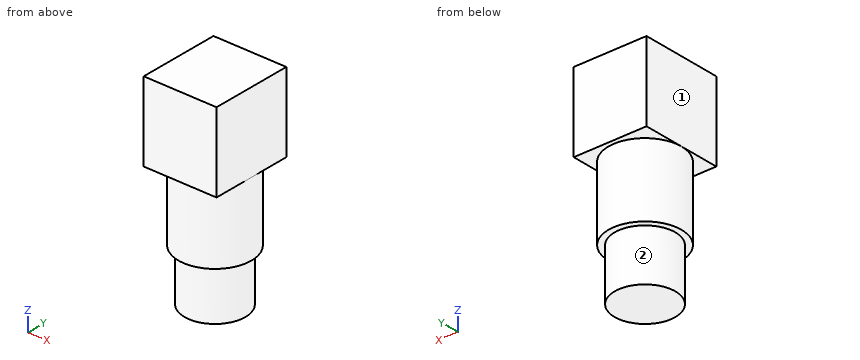
from build123d import *

# Parameters (mm, degrees)
SKETCH003_W             = 12
SKETCH003_H             = 13.4
PAD003_DEPTH            = 13
SKETCH004_R             = 6
PAD004_DEPTH            = 12
SKETCH005_R             = 5
PAD005_DEPTH            = 8.5
BODY002_PLACEMENT_ANGLE = 180


with BuildPart() as part:
    # Sketch003 → Pad003 (new body)
    with BuildSketch(Plane.XY):
        with Locations((6, 6.7)):
            Rectangle(SKETCH003_W, SKETCH003_H)
    extrude(amount=PAD003_DEPTH)

    # Sketch004 (on Face6 of Pad003) → Pad004 (join)
    with BuildSketch(Plane.XY.offset(13)):
        with Locations((6, 6.7)):
            Circle(SKETCH004_R)
    extrude(amount=PAD004_DEPTH)

    # Sketch005 (on Face9 of Pad004) → Pad005 (join)
    with BuildSketch(Plane.XY.offset(25)):
        with Locations((6, 6.7)):
            Circle(SKETCH005_R)
    extrude(amount=PAD005_DEPTH)


with BuildPart() as part_1:
    # Body002 placement: moved
    add(part.part.moved(Location((-6.2, 6.8, -2.4))).rotate(Axis((-6.2, 6.8, -2.4), (1, 0, 0)), BODY002_PLACEMENT_ANGLE))


solid = part_1.part
The model under review builds one solid part; all positions refer to its coordinate system, in mm. Face numbers are marked on the shaded views. A direction names the side the tool comes from. Round coordinates to 2 decimals unless told otherwise and drop trailing zeros. Loops run counter-clockwise (first coordinate to the right, second up) from the corner with the lowest first, then second, coordinate; pieces in that order, holes last. Notation, with made-up numbers: M 57,-8 L 63,-8 A7 cw 63,-4 Z; hole C 44.5,45.25 d8. An arc over 180 degrees is marked long. Answer as a JSON object with one key per item and string values.
Item 1: For line 1 along Z through (x, y) = (-4, 4); line 2 along Z through (x, y) = (-4.25, -6); line 3 along X through (y, z) = (2.5, -25), list the stretches that pass through material, from the lowest coordinate up.
Check sheet entries:
{"line 1": "-27.4 to -2.4", "line 2": "-15.4 to -2.4", "line 3": "-5.7 to 5.3"}
Item 2: We need section A-A, the plane x = -0.2. State the section outline as (y, z) points, and give its area (3 significant figures).
Check sheet entries:
{"outline": "M -6.6,-15.4 L -5.9,-15.4 L -5.9,-27.4 L -4.9,-27.4 L -4.9,-35.9 L 5.1,-35.9 L 5.1,-27.4 L 6.1,-27.4 L 6.1,-15.4 L 6.8,-15.4 L 6.8,-2.4 L -6.6,-2.4 Z", "area": "403 mm2"}
Item 3: We need section B-B, the plane y = 1.25. State the section outline as (x, z) points, and give its area (3 significant figures).
Check sheet entries:
{"outline": "M -6.2,-15.4 L -6.09,-15.4 L -6.09,-27.4 L -5.07,-27.4 L -5.07,-35.9 L 4.67,-35.9 L 4.67,-27.4 L 5.69,-27.4 L 5.69,-15.4 L 5.8,-15.4 L 5.8,-2.4 L -6.2,-2.4 Z", "area": "380 mm2"}
Item 4: We need section C-C, the plane z = -31.5. State the section outline as (x, y) points, and give its area (3 significant figures).
Check sheet entries:
{"outline": "C -0.2,0.1 d10", "area": "78.5 mm2"}
Item 5: Clearance check with flat-ended pins moving along their axes: P1, Ø1.5, axis at y = 3.5, z = -28, coming from the +X side; P2, Ø3, axis at y = 2, z = -19.5, coming from the -X side; P3, Ø1, axis at y = -3.5, z = -22.5, coming from the -X side; P4, Ø3.5, axis at x = -1.5, y = -5, coming from the -Z side. State where each tip first meets the part, or that it passes through.
Check sheet entries:
{"P1": "x = 5.02", "P2": "x = -6.19", "P3": "x = -5.34", "P4": "z = -35.9"}
Item 6: We need section D-D, the plane z = -16. State the section outline as (x, y) points, and give its area (3 significant figures).
Check sheet entries:
{"outline": "C -0.2,0.1 d12", "area": "113 mm2"}
Item 7: Tool access review of the marked faces 1 and 2: name each direction out of +Z, -Z, +X, -X, +Y, -Y from which nothing blocks a thin tool from reaching the whole face with its end or side.
Check sheet entries:
{"face 1": "+Z, -Z, -X, +Y, -Y", "face 2": "-Z"}
